Model file for the job. Use its own axes, mm. Face numbers are marked on the shaded views. A direction names the side the tool comes from. Coordinates: 2 decimals unless noted, no trailing zeros. Write each loop counter-clockwise with the first axis right and the second up, starting at its lowest first coordinate (ties: lowest second). Pieces come first, ordered by that corner, then holes. Notation, with made-up numbers: (79.25, 82.5) -> (114.25, 82.5) arc R30 cw to (114.25, 114.5) -> close; hole circle Ø5 at (67.25, -29.5). An arc over 180 degrees is marked (long way). Write item = value, one per line. Start each with the question number.
from build123d import *

# Parameters (mm, degrees)
SKETCH1_W           = 39.5
SKETCH1_H           = 24.5
BOSS_EXTRUDE1_DEPTH = 40
SKETCH2_W           = 53
SKETCH2_H           = 24.5
BOSS_EXTRUDE2_DEPTH = 2
SKETCH3_R           = 2.25
CUT_EXTRUDE1_DEPTH  = 2
SKETCH4_R           = 2.5
BOSS_EXTRUDE3_DEPTH = 3
SKETCH5_R           = 10.033
BOSS_EXTRUDE4_DEPTH = 1


with BuildPart() as part:
    # Sketch1 → Boss-Extrude1 (new body)
    with BuildSketch(Plane(origin=(0, 0, 0), x_dir=(1, 0, 0), z_dir=(0, 1, 0))):
        Rectangle(SKETCH1_W, SKETCH1_H)
    extrude(amount=BOSS_EXTRUDE1_DEPTH)

    # Sketch2 → Boss-Extrude2 (add)
    with BuildSketch(Plane(origin=(0, 27.5, 0), x_dir=(1, 0, 0), z_dir=(0, 1, 0))):
        Rectangle(SKETCH2_W, SKETCH2_H)
    extrude(amount=-BOSS_EXTRUDE2_DEPTH)

    # Sketch3 → Cut-Extrude1 (cut)
    with BuildSketch(Plane(origin=(0, 27.5, 0), x_dir=(1, 0, 0), z_dir=(0, 1, 0))):
        with Locations(Location((-23.814, 3.752, 0), (0, 0, 270))):
            Circle(SKETCH3_R)
        with Locations(Location((-23.814, -6.154, 0), (0, 0, 270))):
            Circle(SKETCH3_R)
        with Locations(Location((23.814, 3.752, 0), (0, 0, 270))):
            Circle(SKETCH3_R)
        with Locations(Location((23.814, -6.154, 0), (0, 0, 270))):
            Circle(SKETCH3_R)
    extrude(amount=-CUT_EXTRUDE1_DEPTH, mode=Mode.SUBTRACT)

    # Sketch4 → Boss-Extrude3 (add)
    with BuildSketch(Plane(origin=(0, 40, 0), x_dir=(1, 0, 0), z_dir=(0, 1, 0))):
        with Locations(Location((-9.25, -1.75, 0), (0, 0, 270))):
            Circle(SKETCH4_R)
    extrude(amount=BOSS_EXTRUDE3_DEPTH)

    # Sketch5 → Boss-Extrude4 (add)
    with BuildSketch(Plane(origin=(0, 43, 0), x_dir=(1, 0, 0), z_dir=(0, 1, 0))):
        with Locations(Location((-9.25, -1.75, 0), (0, 0, 270))):
            Circle(SKETCH5_R)
    extrude(amount=BOSS_EXTRUDE4_DEPTH)


solid = part.part
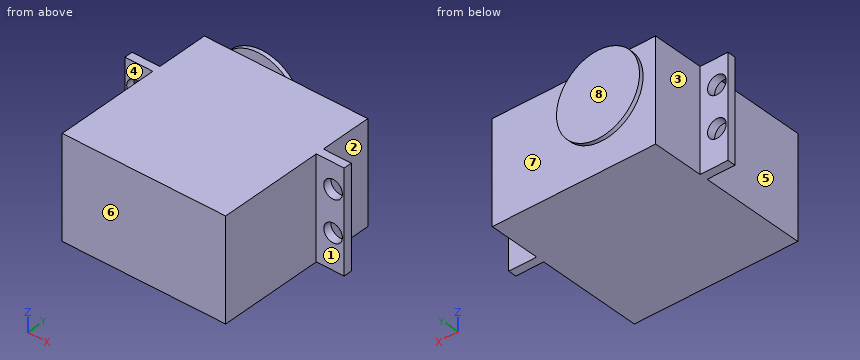
(1) Saw through at D-D (z = 1.75). Give the cut face in (x, y).
(2) Saw through at A-A (z = -4). Give the cut face in (x, y), then the cut area to 3 significant figures.
(3) Drill centre lines: line 1 along X through (y, z) = (7, 4); line 2 along Y through (x, z) = (13.5, 1.25); line 3 along Y through (x, z) = (-6, -0.5). Where is each one in solid material? Low to high.
(4) Mould opens along Y. For the marked faces 5, 6, 7 and 8 say: released by +Y, released by -Y, zero draft, split by the parting line, or undercut.
(5) Saw through at B-B (x = -9.25). Give the cut face in (y, z).
(6) Saw through at C-C (x = -0.5). Give the cut face in (y, z).
(7) 3-axis set-ups, long thin cutter, end or side, ignore diameter. For the marked faces 1, 2, 3 and 4: which of +Z, -Z, +X, -X, +Y, -Y reach the whole face in a straight line?
(8) Drop flat-ended pins along their axis: pin 1 Ø5.5 at (x, z) = (23.5, -5) entering from +Y; pin 2 Ø6 at (y, z) = (32.5, 1.5) entering from -X; pin 3 Ø4 at (y, z) = (31, -2) entering from +X; pin 4 Ø4 at (x, z) = (23.814, -3.752) entering from +Y (3 decimals). Give the stop position or say it passes through.
Returned:
q1.outline = (-26.5, 25.5) -> (-19.75, 25.5) -> (-19.75, 0) -> (19.75, 0) -> (19.75, 25.5) -> (26.5, 25.5) -> (26.5, 27.5) -> (19.75, 27.5) -> (19.75, 40) -> (-6.75, 40) -> (-6.75, 43) -> (0.78, 43) -> (0.78, 44) -> (-19.28, 44) -> (-19.28, 43) -> (-11.75, 43) -> (-11.75, 40) -> (-19.75, 40) -> (-19.75, 27.5) -> (-26.5, 27.5) -> close
q2.outline = (-26.5, 25.5) -> (-26.05, 25.5) -> (-26.05, 27.5) -> (-26.5, 27.5) -> close; (-21.58, 25.5) -> (-19.75, 25.5) -> (-19.75, 0) -> (19.75, 0) -> (19.75, 25.5) -> (21.58, 25.5) -> (21.58, 27.5) -> (19.75, 27.5) -> (19.75, 40) -> (-19.75, 40) -> (-19.75, 27.5) -> (-21.58, 27.5) -> close; (-17.47, 43) -> (-1.03, 43) -> (-1.03, 44) -> (-17.47, 44) -> close; (26.05, 25.5) -> (26.5, 25.5) -> (26.5, 27.5) -> (26.05, 27.5) -> close
q2.area = 1,610 mm2
q3.line_1 = -19.75 to 19.75
q3.line_2 = 0 to 40
q3.line_3 = 0 to 40, 43 to 44
q4.face_5 = zero draft
q4.face_6 = released by -Y
q4.face_7 = undercut
q4.face_8 = released by +Y
q5.outline = (0, -12.25) -> (40, -12.25) -> (40, -0.75) -> (43, -0.75) -> (43, -8.28) -> (44, -8.28) -> (44, 11.78) -> (43, 11.78) -> (43, 4.25) -> (40, 4.25) -> (40, 12.25) -> (0, 12.25) -> close
q6.outline = (0, -12.25) -> (40, -12.25) -> (40, 12.25) -> (0, 12.25) -> close; (43, -3.16) -> (44, -3.16) -> (44, 6.66) -> (43, 6.66) -> close
q7.face_1 = +Z, -Z, +X, -Y
q7.face_2 = +Z, -Z, +X, +Y
q7.face_3 = +Z, -Z, -X, +Y
q7.face_4 = +Z, -Z, -X, -Y
q8.pin_1 = 27.5
q8.pin_2 = -19.75
q8.pin_3 = 19.75
q8.pin_4 = through
